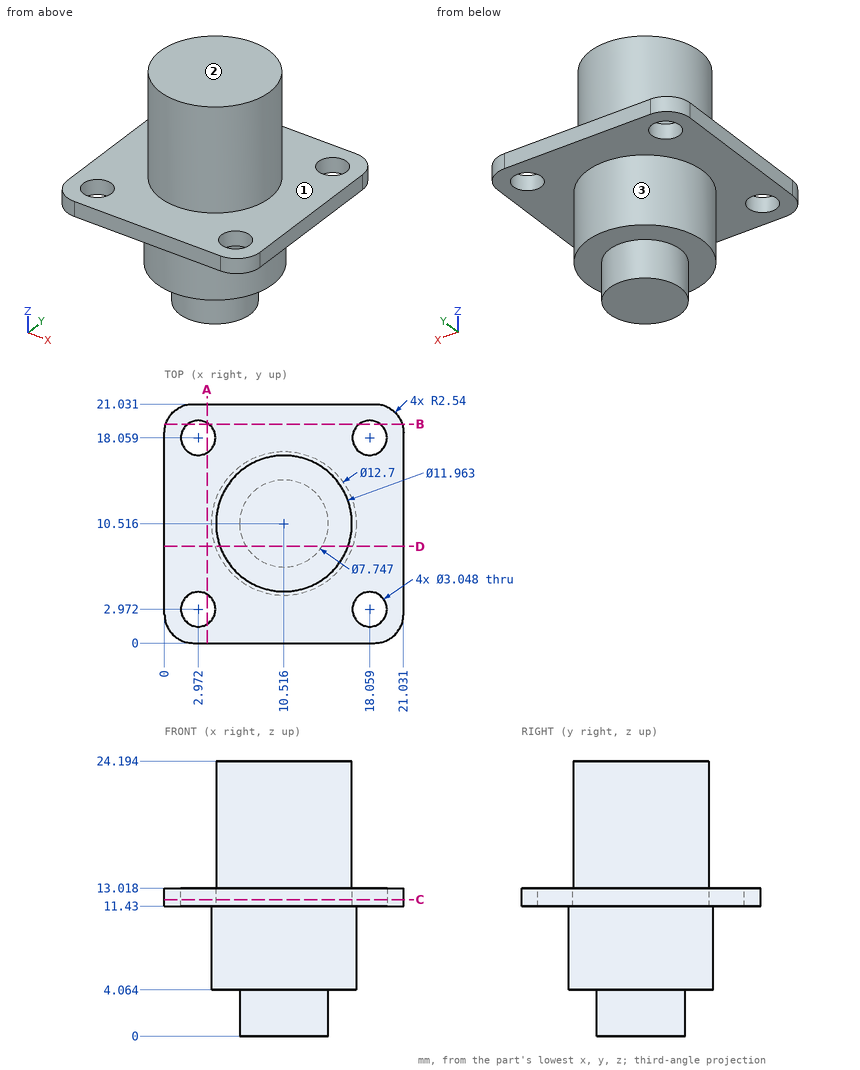
Could you check a few things on this drawing? It's one solid part, dimensions in mm from its lowest x, y, z. A direction names the side the tool comes from. Give positions to 0.01 mm unless a question says otherwise; leave off trailing zeros. Order: outer loops, then holes, each group sorted by start corner. A loop starts at its lowest first (then second) coordinate and runs counter-clockwise, first axis right, second up. Notation, with made-up numbers: (38, 13) -> (64, 13) arc R16 cw to (64, 30) -> close; hole circle Ø3 at (10, 32). An arc over 180 degrees is marked (long way). Answer in a Markdown table with one row per item. Add a question column.
Item 1: Imagine slicing it at A-A (x = 3.75). List the corners of the cut face in (y, z) for me.
Item 2: Please list where these lines run through material, in increasing order: probe 1 along Y at (x, z) = (10.5, 21); probe 2 along Z at (x, y) = (8.75, 6.75) (1 decimal); probe 3 along Z at (x, y) = (15.25, 18.75).
Item 3: For the marked faces 1, 2 and 3, which set-ups out of +Z, -Z, +X, -X, +Y, -Y let a thin tool reach every point of the face, with its end or its side?
Item 4: I'm going to push flat-ended pins straight in: P1, Ø2, axis at y = 12, z = 4, coming from the -X side; P2, Ø2.5, axis at x = 18.06, y = 18.06, coming from the +Z side; P3, Ø4, axis at x = 11, z = 7, coming from the -Y side; P4, Ø1.5, axis at y = 12.5, z = 16.5, coming from the +X side. Where does each tip first touch, or does it pass through?
Item 5: Imagine slicing it at C-C (z = 12). List the corners of the cut face in (x, y) for me (1 decimal).
Item 6: Imagine slicing it at B-B (y = 19.25). List the corners of the cut face in (x, z) for me (1 decimal).
Item 7: Imagine slicing it at D-D (y = 8.5). List the corners of the cut face in (x, z) for me (1 decimal), and give its area (3 significant figures).
Result:
| question | item | result |
|---|---|---|
| 1 | outline | (0, 11.43) -> (1.66, 11.43) -> (1.66, 13.02) -> (0, 13.02) -> close; (4.28, 11.43) -> (16.75, 11.43) -> (16.75, 13.02) -> (4.28, 13.02) -> close; (19.37, 11.43) -> (21.03, 11.43) -> (21.03, 13.02) -> (19.37, 13.02) -> close |
| 2 | probe 1 | 4.53 to 16.5 |
| 2 | probe 2 | 4.1 to 24.2 |
| 2 | probe 3 | 11.43 to 13.02 |
| 3 | face 1 | +Z |
| 3 | face 2 | +Z, +X, -X, +Y, -Y |
| 3 | face 3 | -Z |
| 4 | P1 | x = 4.18 |
| 4 | P2 | through |
| 4 | P3 | y = 4.17 |
| 4 | P4 | x = 16.37 |
| 5 | outline | (0, 2.5) arc R2.5 ccw to (2.5, 0) -> (18.5, 0) arc R2.5 ccw to (21, 2.5) -> (21, 18.5) arc R2.5 ccw to (18.5, 21) -> (2.5, 21) arc R2.5 ccw to (0, 18.5) -> close; hole circle Ø3 at (3, 3); hole circle Ø3 at (3, 18.1); hole circle Ø3 at (18.1, 3); hole circle Ø3 at (18.1, 18.1) |
| 6 | outline | (0.1, 11.4) -> (2, 11.4) -> (2, 13) -> (0.1, 13) -> close; (3.9, 11.4) -> (17.1, 11.4) -> (17.1, 13) -> (3.9, 13) -> close; (19, 11.4) -> (20.9, 11.4) -> (20.9, 13) -> (19, 13) -> close |
| 7 | outline | (0, 11.4) -> (4.5, 11.4) -> (4.5, 4.1) -> (7.2, 4.1) -> (7.2, 0) -> (13.8, 0) -> (13.8, 4.1) -> (16.5, 4.1) -> (16.5, 11.4) -> (21, 11.4) -> (21, 13) -> (16.1, 13) -> (16.1, 24.2) -> (4.9, 24.2) -> (4.9, 13) -> (0, 13) -> close |
| 7 | area | 275 mm2 |
